For this review, use the dimensioned drawing (mm, ordinates from the lowest corner) and the shaded views. A direction names the side the tool comes from. Give positions to 0.01 mm unless a question says otherwise; leave off trailing zeros. Loops run counter-clockwise (first coordinate to the right, second up) from the corner with the lowest first, then second, coordinate; pieces in that order, holes last. Notation, with made-up numbers: M 17.25,31 L 24.25,31 A24 cw 24.25,51 Z; hole C 76.5,-5.5 d4. An arc over 180 degrees is marked long. Return JSON: item names as keys, results as strings.
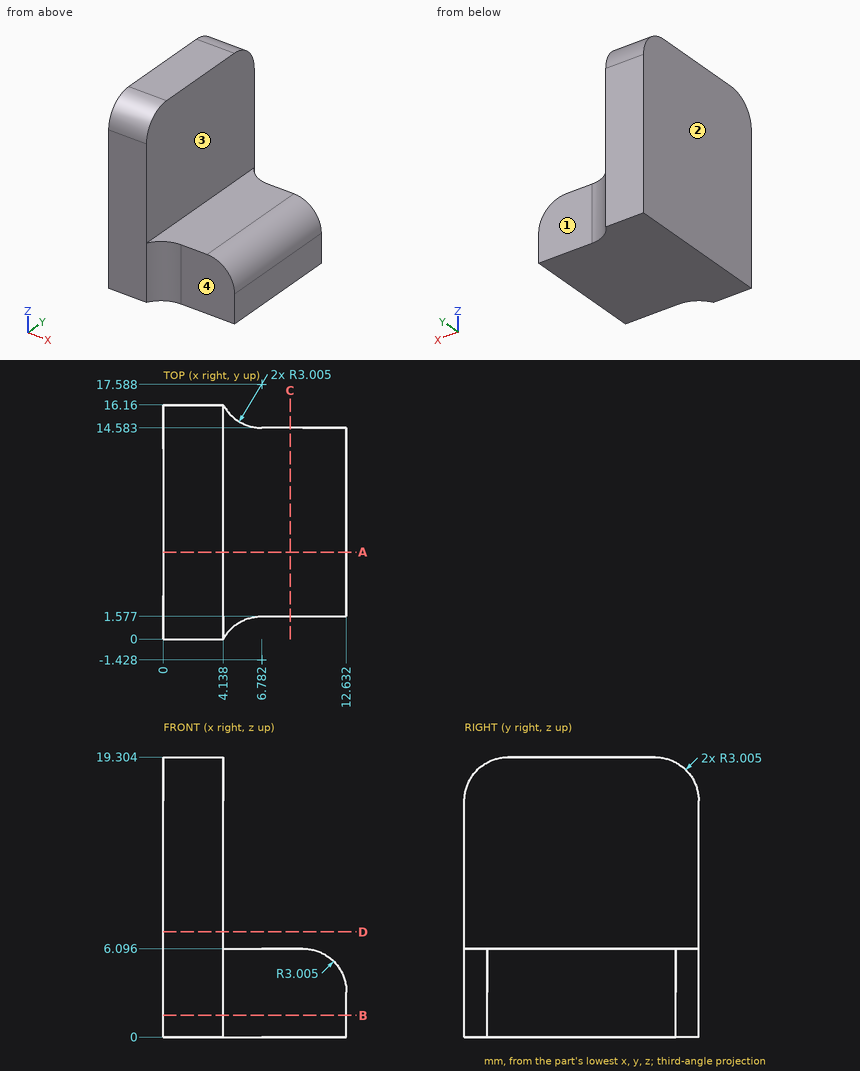
1) Consider section B-B on z = 1.5. Write out the cut boundary in (x, y) (1 decimal).
From the geometry:
{"outline": "M 0,0 L 4.1,0 A3 cw 6.8,1.6 L 12.6,1.6 L 12.6,14.6 L 6.8,14.6 A3 cw 4.1,16.2 L 0,16.2 Z"}
2) Consider section A-A on y = 6. Write out the cut boundary in (x, z) (1 decimal).
From the geometry:
{"outline": "M 0,0 L 12.6,0 L 12.6,3.1 A3 ccw 9.6,6.1 L 4.1,6.1 L 4.1,19.3 L 0,19.3 Z"}
3) Consider section C-C on x = 8.75. Write out the cut boundary in (y, z).
From the geometry:
{"outline": "M 1.58,0 L 14.58,0 L 14.58,6.1 L 1.58,6.1 Z"}
4) Wall thickness on L1, parallel to Y at x = 7, z = 5.5; L2, parallel to Z at x = 6.5, y = 12; L3, parallel to X at y = 13.75, z = 10: over which ranges is each line inside the solid? List them lowest first. Write a range as from..to.
From the geometry:
{"L1": "1.58..14.58", "L2": "0..6.1", "L3": "0..4.14"}
5) Tool access review of the marked faces 1, 2, 3 and 4: name each direction out of +Z, -Z, +X, -X, +Y, -Y from which nothing blocks a thin tool from reaching the whole face with its end or side.
From the geometry:
{"face 1": "+Z, -Z, +X, +Y", "face 2": "+Z, -Z, -X, +Y, -Y", "face 3": "+Z, +X, +Y, -Y", "face 4": "+Z, -Z, +X, -Y"}
6) Consider section D-D on z = 7.25. Write out the cut boundary in (x, y).
From the geometry:
{"outline": "M 0,0 L 4.14,0 L 4.14,16.16 L 0,16.16 Z"}
7) Insertion check: pin 1 (1.5 mm diameter, centred on x = 10, z = 3.5, fed in from -Y); pin 2 (2.5 mm diameter, centred on x = 7, y = 5, fed in from +Z); pin 3 (4 mm diameter, centred on y = 7.5, z = 13, fed in from +X). Each pin has a flat end and moves straight along its axis. Give the tip position at first contact, or say it passes through.
From the geometry:
{"pin 1": "y = 1.58", "pin 2": "z = 6.1", "pin 3": "x = 4.14"}
